```python
from build123d import *

# Parameters (mm, degrees)
F0_R      = 14.9225
F1_DEPTH  = 7.62
F2_R      = 11.0236
F3_DEPTH  = 25.4
F5_DEPTH  = 7.62
F6_DEPTH  = 7.62
F7_R      = 14.9225
F8_DEPTH  = 7.62
F9_R      = 11.0236
F10_DEPTH = 25.4


with BuildPart() as f1:
    # F0 (on Top) → F1 (new body)
    with BuildSketch(Plane.XY):
        Circle(F0_R)
    extrude(amount=F1_DEPTH)

    # F2 (on face) → F3 (cut)
    with BuildSketch(Plane.XY.offset(7.62)):
        Circle(F2_R)
    extrude(amount=-F3_DEPTH, mode=Mode.SUBTRACT)

    # F4 (on Top) → F5 (join)
    with BuildSketch(Plane.XY):
        with BuildLine():
            Line((2.708977, 33.321824), (-3.027178, 34.026534))
            ThreePointArc((-3.027178, 34.026534), (-5.061644, 23.760928), (-0.211553, 14.487399))
            Line((-0.211553, 14.487399), (5.524602, 13.782689))
            ThreePointArc((5.524602, 13.782689), (0.674511, 23.056218), (2.708977, 33.321824))
        make_face()
        with BuildLine():
            Line((0.229531, -34.11213), (6.113042, -34.834943))
            ThreePointArc((6.113042, -34.834943), (7.902941, -24.423116), (2.708977, -15.223516))
            Line((2.708977, -15.223516), (-4.207222, -14.373833))
            ThreePointArc((-4.207222, -14.373833), (1.600579, -23.436154), (0.229531, -34.11213))
        make_face()
    extrude(amount=F5_DEPTH)

    # F4 (on Top) → F6 (join)
    with BuildSketch(Plane.XY):
        with BuildLine():
            Line((2.708977, 33.321824), (-3.027178, 34.026534))
            ThreePointArc((-3.027178, 34.026534), (-5.061644, 23.760928), (-0.211553, 14.487399))
            Line((-0.211553, 14.487399), (5.524602, 13.782689))
            ThreePointArc((5.524602, 13.782689), (0.674511, 23.056218), (2.708977, 33.321824))
        make_face()
        with BuildLine():
            Line((0.229531, -34.11213), (6.113042, -34.834943))
            ThreePointArc((6.113042, -34.834943), (7.902941, -24.423116), (2.708977, -15.223516))
            Line((2.708977, -15.223516), (-4.207222, -14.373833))
            ThreePointArc((-4.207222, -14.373833), (1.600579, -23.436154), (0.229531, -34.11213))
        make_face()
    extrude(amount=F6_DEPTH)

    # F7 (on Top) → F8 (join)
    with BuildSketch(Plane.XY):
        with Locations((0, 48.594203)):
            Circle(F7_R)
        with Locations((0, -48.849575)):
            Circle(F7_R)
    extrude(amount=F8_DEPTH)

    # F9 (on face) → F10 (cut)
    with BuildSketch(Plane.XY.offset(7.62)):
        with Locations((0, 48.594203)):
            Circle(F9_R)
        with Locations((0, -48.849575)):
            Circle(F9_R)
    extrude(amount=-F10_DEPTH, mode=Mode.SUBTRACT)


solid = f1.part
```
Geometry: final body of the model. Coordinates: model frame, mm. Give positions to 0.01 mm unless a question says otherwise; leave off trailing zeros. Order: outer loops, then holes, each group sorted by start corner. A loop starts at its lowest first (then second) coordinate and runs counter-clockwise, first axis right, second up. Notation, with made-up numbers: (5, -20) -> (13, -20) arc R16 ccw to (13, -10) -> close; hole circle Ø10 at (2, -40). An arc over 180 degrees is marked (long way). Write each question's results on one line, items separated by ' | '. Start each with the question number.
1) Section A-A (y = 0). Return loops of the section in (x, z), then the cut area to 3 significant figures.
2) Section B-B (x = -9.5). Return loops of the section in (y, z), then the cut area to 3 significant figures.
3) Line query: line 1 (Y direction, x = -8.5, z = 3.5); line 2 (Y direction, x = -7, z = 1.25); line 3 (Y direction, x = -12, z = 6.75). Output: solid intervals per line, ascending. Write a range as from..to.
4) Draft query along Y for faces 1 (the cylindrical face through (0.68, 23.01, 3.76)), 2 (the flat face through (-7, -9, 0)). Return one class per face: pulls with the +Y half, pulls with the -Y half, needs draft (parallel to the pull), parting line crosses it, or undercut.
5) First-contact query: pin 1 (1 mm diameter, centred on x = 8.5, z = 5.5, fed in from -Y); pin 2 (1.5 mm diameter, centred on y = -41, z = 5, fed in from -X); pin 3 (8 mm diameter, centred on x = -3.5, y = -2, fed in from +Z); pin 4 (1 mm diameter, centred on x = 6, z = 3.5, fed in from +Y). Flat tips, straight axial feed; report the tip coordinate or a pass-through.
6) Section C-C (y = -39). Return loops of the section in (x, z), then the cut area to 3 significant figures.
Calculated:
1) outline: (-14.92, 0) -> (-11.02, 0) -> (-11.02, 7.62) -> (-14.92, 7.62) -> close; (11.02, 0) -> (14.92, 0) -> (14.92, 7.62) -> (11.02, 7.62) -> close | area: 59.4 mm2
2) outline: (-60.36, 0) -> (-54.44, 0) -> (-54.44, 7.62) -> (-60.36, 7.62) -> close; (-43.26, 0) -> (-37.34, 0) -> (-37.34, 7.62) -> (-43.26, 7.62) -> close; (-11.51, 0) -> (-5.59, 0) -> (-5.59, 7.62) -> (-11.51, 7.62) -> close; (5.59, 0) -> (11.51, 0) -> (11.51, 7.62) -> (5.59, 7.62) -> close; (37.09, 0) -> (43, 0) -> (43, 7.62) -> (37.09, 7.62) -> close; (54.19, 0) -> (60.1, 0) -> (60.1, 7.62) -> (54.19, 7.62) -> close | area: 270 mm2
3) line 1: -61.11..-55.87, -41.83..-36.58, -12.27..-7.02, 7.02..12.27, 36.33..41.57, 55.61..60.86 | line 2: -62.03..-57.37, -40.33..-35.67, -13.18..-8.52, 8.52..13.18, 35.42..40.08, 57.11..61.77 | line 3: -57.72..-39.98, -8.87..8.87, 39.72..57.46
4) face 1: undercut | face 2: needs draft
5) pin 1: y = -61.45 | pin 2: x = -13.13 | pin 3: through | pin 4: y = 62.47
6) outline: (-11.21, 0) -> (-4.95, 0) -> (-4.95, 7.62) -> (-11.21, 7.62) -> close; (4.95, 0) -> (11.21, 0) -> (11.21, 7.62) -> (4.95, 7.62) -> close | area: 95.4 mm2
